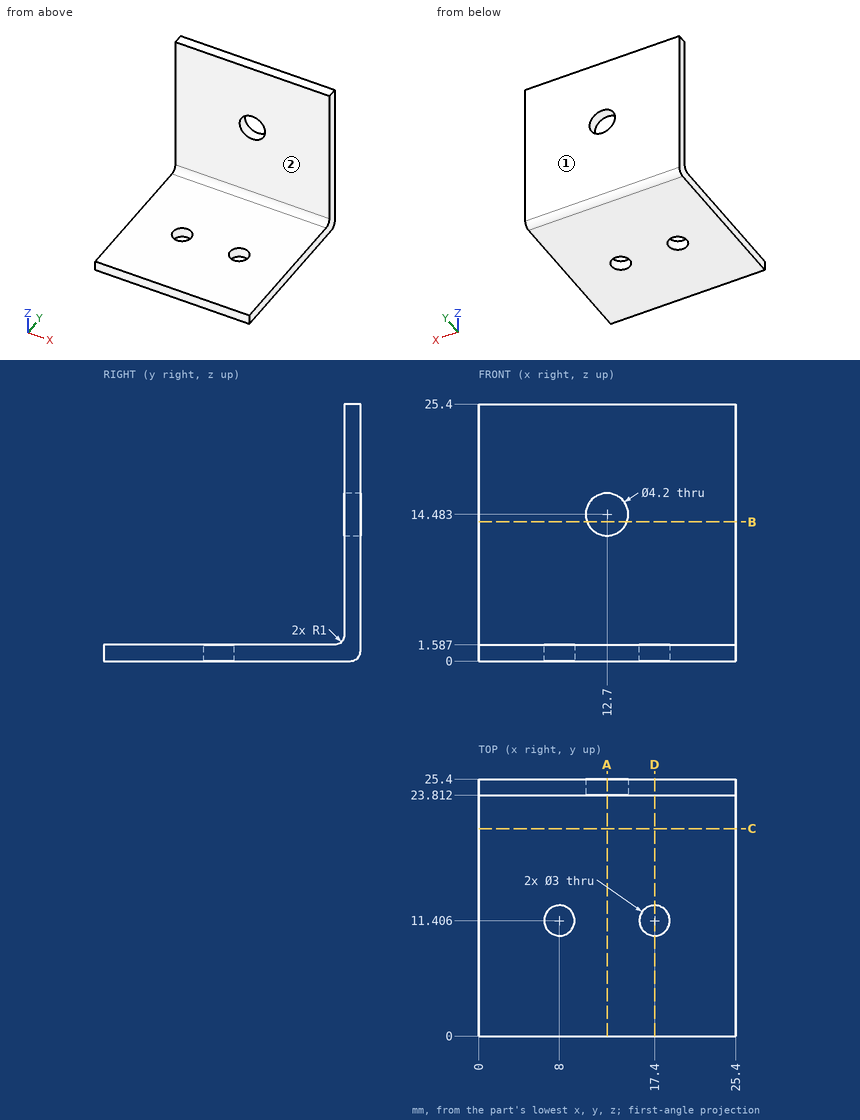
Input: dimensioned drawing with shaded views. Units: mm. Origin: part minimum x, y, z. A direction names the side the tool comes from. Give positions to 0.01 mm unless a question says otherwise; leave off trailing zeros. Write each loop counter-clockwise with the first axis right and the second up, starting at its lowest first coordinate (ties: lowest second). Pieces come first, ordered by that corner, then holes. Notation, with made-up numbers: (7, 53) - (27, 53) arc R18 cw to (27, 66) - close; hole circle Ø5 at (72.25, -29.75). An arc over 180 degrees is marked (long way). One line per item, written item: value. Start each with the question number.
Q1. First-contact query: pin 1 Ø1.8 at (x, y) = (17.4, 11.41) entering from -Z; pin 2 Ø3.5 at (x, y) = (8, 11.41) entering from +Z; pin 3 Ø5 at (x, z) = (10, 17.5) entering from -Y. Flat tips, straight axial feed; report the tip coordinate or a pass-through.
Q2. Set-up query: the marked faces 1 and 2. Return all of +Z, -Z, +X, -X, +Y, -Y with unobstructed straight access to the full face (end or side cutting, diameter ignored); none if empty.
Q3. Section query A-A, the plane x = 12.7. Return the cut outline in (y, z).
Q4. Section query C-C, the plane y = 20.5. Return the cut outline in (x, z).
Q5. Material intervals for probe 1 along Y at (x, z) = (17.4, 0.9) (1 decimal); probe 2 along Y at (x, z) = (15.75, 10); probe 3 along Z at (x, y) = (5, 11.5), sorted ascending. Write a range as from..to.
Q6. Section query D-D, the plane x = 17.4. Return the cut outline in (y, z).
Q7. Section query B-B, the plane z = 13.75. Return the cut outline in (x, y).
Answer:
1. pin 1: passes through
1. pin 2: stops at z = 1.59
1. pin 3: stops at y = 23.81
2. face 1: +Z, -Z, +X, -X, +Y
2. face 2: +Z, +X, -X, -Y
3. outline: (0, 0) - (24.4, 0) arc R1 ccw to (25.4, 1) - (25.4, 12.38) - (23.81, 12.38) - (23.81, 2.59) arc R1 cw to (22.81, 1.59) - (0, 1.59) - close; (23.81, 16.58) - (25.4, 16.58) - (25.4, 25.4) - (23.81, 25.4) - close
4. outline: (0, 0) - (25.4, 0) - (25.4, 1.59) - (0, 1.59) - close
5. probe 1: y = 0..9.9, 12.9..25.4
5. probe 2: y = 23.81..25.4
5. probe 3: z = 0..1.59
6. outline: (0, 0) - (9.91, 0) - (9.91, 1.59) - (0, 1.59) - close; (12.91, 0) - (24.4, 0) arc R1 ccw to (25.4, 1) - (25.4, 25.4) - (23.81, 25.4) - (23.81, 2.59) arc R1 cw to (22.81, 1.59) - (12.91, 1.59) - close
7. outline: (0, 23.81) - (10.73, 23.81) - (10.73, 25.4) - (0, 25.4) - close; (14.67, 23.81) - (25.4, 23.81) - (25.4, 25.4) - (14.67, 25.4) - close
